Here's how the part is built. I have some questions about the finished solid (model axes, mm). Give positions to 0.01 mm unless a question says otherwise; leave off trailing zeros. Loops run counter-clockwise (first coordinate to the right, second up) from the corner with the lowest first, then second, coordinate; pieces in that order, holes last.
Q1. If we section it at D-D (x = 31.5): Please give me the cut outline in (y, z), plus the area to 3 significant figures.
Q2. If we section it at A-A (x = 12.5): Please give me the cut outline in (y, z), plus the area to 3 significant figures.
Q3. We'd pull the mould along X, two halves only. Please class faces 1 (the face through (-3.922, -1.503, 102.477)), 2 (the face through (-11.795, -1.503, 30.681)), 3 (the face through (-0.28, -1.5, 123.82)), 4 (the face through (3, -3.048, 59)): +X half, -X half, draft (parallel to the pull), parting line (faces both ways), or undercut.
Q4. If we section it at B-B (y = -2.05): Give the number of separate pieces and of enclosed holes in the cut face, plus the area to 3 significant figures.
Q5. Will these pins go through, and if not, where does the flat tip stop? P1, Ø1.5, axis at y = -2.5, z = 5.5, coming from the -X side; P2, Ø1.5, axis at x = 19.5, y = -1.5, coming from the +Z side.
Q6. I need wall thicknesses on line 1 (Z direction, x = 0, y = -0.7) (3 decimals); line 2 (Z direction, x = 37, y = -2.5); line 3 (X direction, y = -2.1, z = 114.3). Which ranges of each line are inside material? Lowest first, please.
Q7. If we section it at C-C (z = 44.5): Please give me the cut outline in (x, y).
from build123d import *

# Parameters (mm, degrees)
F0_R     = 2.2225
F1_DEPTH = 3.048


# Not quite as in the source:
# - ends of sketch curves that miss each other by under 0.0002 mm in the source are joined


with BuildPart() as f1:
    # F0 (on Front) → F1 (new body)
    with BuildSketch(Plane.XZ):
        with BuildLine():
            Line((0, 104.775), (0, 79.375))
            ThreePointArc((0, 79.375), (9.9062001273, 75.9049515935), (15.4816923534, 67.0118124772))
            ThreePointArc((15.4816923534, 67.0118124772), (15.634754331, 66.2513782015), (15.7504882737, 65.484375))
            Line((15.7504882737, 65.484375), (9.4502929642, 115.490625))
            ThreePointArc((9.4502929642, 115.490625), (9.5063048942, 114.896483242), (9.525, 114.3))
            ThreePointArc((9.525, 114.3), (6.7351920908, 107.5648079092), (0, 104.775))
        make_face()
        with BuildLine():
            ThreePointArc((-15.3768101201, 67.4457997325), (-9.7307773134, 76.0430298523), (0, 79.375))
            Line((0, 79.375), (0, 104.775))
            ThreePointArc((0, 104.775), (-6.8164586923, 107.6470671207), (-9.5221925783, 114.5312433813))
            Line((-9.5221925783, 114.5312433813), (-15.3768101201, 67.4457997325))
        make_face()
        with Locations((-3.6322334781, 100.2735868096)):
            Circle(F0_R, mode=Mode.SUBTRACT)
        with BuildLine():
            ThreePointArc((-9.5221925783, 114.5312433813), (-6.8164586923, 107.6470671207), (0, 104.775))
            ThreePointArc((0, 104.775), (6.7351920908, 107.5648079092), (9.525, 114.3))
            ThreePointArc((9.525, 114.3), (9.5063048942, 114.896483242), (9.4502929642, 115.490625))
            ThreePointArc((9.4502929642, 115.490625), (-0.481036029, 123.8128454912), (-9.5221925783, 114.5312433813))
        make_face()
        with BuildLine():
            ThreePointArc((3.1731383542, 114.3), (2.2437476479, 112.0562523521), (0, 111.1268616458))
            ThreePointArc((0, 111.1268616458), (-2.2437476479, 116.5437476479), (3.1731383542, 114.3))
        make_face(mode=Mode.SUBTRACT)
        with BuildLine():
            Line((0, 59.2630050683), (0, 47.625))
            ThreePointArc((0, 47.625), (9.5420870367, 50.8128332563), (15.2519117252, 59.0960456714))
            Line((15.2519117252, 59.0960456714), (15.8668198703, 64.0095607934))
            Line((15.8668198703, 64.0095607934), (15.4816923534, 67.0118124772))
            ThreePointArc((15.4816923534, 67.0118124772), (9.9062001273, 75.9049515935), (0, 79.375))
            Line((0, 79.375), (0, 67.7369949317))
            ThreePointArc((0, 67.7369949317), (2.996007848, 66.496007848), (4.2369949317, 63.5))
            ThreePointArc((4.2369949317, 63.5), (2.996007848, 60.503992152), (0, 59.2630050683))
        make_face()
        with BuildLine():
            ThreePointArc((-15.7459735632, 61.4801134818), (-10.4868948341, 51.5819187057), (0, 47.625))
            Line((0, 47.625), (0, 59.2630050683))
            ThreePointArc((0, 59.2630050683), (-4.2369949317, 63.5), (0, 67.7369949317))
            Line((0, 67.7369949317), (0, 79.375))
            ThreePointArc((0, 79.375), (-9.7307773134, 76.0430298523), (-15.3768101201, 67.4457997325))
            Line((-15.3768101201, 67.4457997325), (-15.8748867846, 63.4400452066))
            ThreePointArc((-15.8748867846, 63.4400452066), (-15.8407712999, 62.4580836766), (-15.7459735632, 61.4801134818))
        make_face()
        with BuildLine():
            ThreePointArc((-7.7320952095, -0.9918697506), (-5.8524002287, 5.1496129461), (0, 7.7954539272))
            Line((0, 7.7954539272), (0, 47.625))
            ThreePointArc((0, 47.625), (-10.4868948341, 51.5819187057), (-15.7459735632, 61.4801134818))
            Line((-15.7459735632, 61.4801134818), (-7.7320952095, -0.9918697506))
        make_face()
        with BuildLine():
            Line((0, 47.625), (0, 7.7954539272))
            ThreePointArc((0, 7.7954539272), (5.5122183343, 5.5122183343), (7.7954539272, 0))
            Line((7.7954539272, 0), (36.5125, 0))
            ThreePointArc((36.5125, 0), (38.6941635505, 5.4657344444), (44.0398708389, 7.9268972695))
            Line((44.0398708389, 7.9268972695), (17.869380753, 7.8488082918))
            ThreePointArc((17.869380753, 7.8488082918), (11.8930439791, 10.5290526777), (9.9569931381, 16.7862100471))
            Line((9.9569931381, 16.7862100471), (15.2519117252, 59.0960456714))
            ThreePointArc((15.2519117252, 59.0960456714), (9.5420870367, 50.8128332563), (0, 47.625))
        make_face()
        with BuildLine():
            Line((36.5125, 0), (7.7954539272, 0))
            ThreePointArc((7.7954539272, 0), (5.5122183343, -5.5122183343), (0, -7.7954539272))
            Line((0, -7.7954539272), (43.9269950713, -7.9202507596))
            ThreePointArc((43.9269950713, -7.9202507596), (38.6553793104, -5.4245992768), (36.5125, 0))
        make_face()
        with BuildLine():
            ThreePointArc((3.0872431229, 0), (-2.1830105474, -2.1830105474), (0, 3.0872431229))
            Line((0, 3.0872431229), (0, 7.7954539272))
            ThreePointArc((0, 7.7954539272), (-5.8524002287, 5.1496129461), (-7.7320952095, -0.9918697506))
            ThreePointArc((-7.7320952095, -0.9918697506), (-5.1496129461, -5.8524002287), (0, -7.7954539272))
            ThreePointArc((0, -7.7954539272), (5.5122183343, -5.5122183343), (7.7954539272, 0))
            Line((7.7954539272, 0), (3.0872431229, 0))
        make_face()
        with BuildLine():
            Line((0, 7.7954539272), (0, 3.0872431229))
            ThreePointArc((0, 3.0872431229), (2.1830105474, 2.1830105474), (3.0872431229, 0))
            Line((3.0872431229, 0), (7.7954539272, 0))
            ThreePointArc((7.7954539272, 0), (5.5122183343, 5.5122183343), (0, 7.7954539272))
        make_face()
        with BuildLine():
            ThreePointArc((44.0398708389, 7.9268972695), (38.6941635505, 5.4657344444), (36.5125, 0))
            ThreePointArc((36.5125, 0), (38.6553793104, -5.4245992768), (43.9269950713, -7.9202507596))
            Line((43.9269950713, -7.9202507596), (44.9280052412, -7.9230939184))
            ThreePointArc((44.9280052412, -7.9230939184), (50.2291899455, -5.4410357308), (52.3875, 0))
            ThreePointArc((52.3875, 0), (49.9157344444, 5.7558364495), (44.0398708389, 7.9268972695))
        make_face()
        with BuildLine():
            ThreePointArc((47.2789731749, 0), (44.45, -2.8289731749), (41.6210268251, 0))
            ThreePointArc((41.6210268251, 0), (44.45, 2.8289731749), (47.2789731749, 0))
        make_face(mode=Mode.SUBTRACT)
    extrude(amount=F1_DEPTH)


solid = f1.part
Check sheet entries:
1. outline: (-3.05, -7.88) - (0, -7.88) - (0, 7.89) - (-3.05, 7.89) - close
1. area: 48.1 mm2
2. outline: (-3.05, -7.83) - (0, -7.83) - (0, 9.91) - (-3.05, 9.91) - close; (-3.05, 37.11) - (0, 37.11) - (0, 91.28) - (-3.05, 91.28) - close
2. area: 219 mm2
3. face 1: undercut
3. face 2: -X half
3. face 3: parting line
3. face 4: draft
4. separate pieces: 1
4. enclosed holes: 5
4. area: 3,590 mm2
5. P1: stops at x = -8.66
5. P2: stops at z = 7.86
6. line 1: z = -7.795 to -3.087, 3.087 to 59.263, 67.737 to 111.127, 117.473 to 123.825
6. line 2: z = -7.9 to 7.91
6. line 3: x = -9.55 to -3.17, 3.17 to 9.6
7. outline: (-13.57, -3.05) - (13.43, -3.05) - (13.43, 0) - (-13.57, 0) - close
